Design review of the part built by this model. Coordinates are the model's own, in mm. Face numbers are marked on the shaded views. Give positions to 0.01 mm unless a question says otherwise; leave off trailing zeros. Write each loop counter-clockwise with the first axis right and the second up, starting at its lowest first coordinate (ties: lowest second). Pieces come first, ordered by that corner, then holes. Notation, with made-up numbers: M 45,8 L 73,8 A21 ccw 73,44 Z; hole C 17.5,36 d3. An arc over 180 degrees is marked long. Use a Markdown table: item, result. Add a question column.
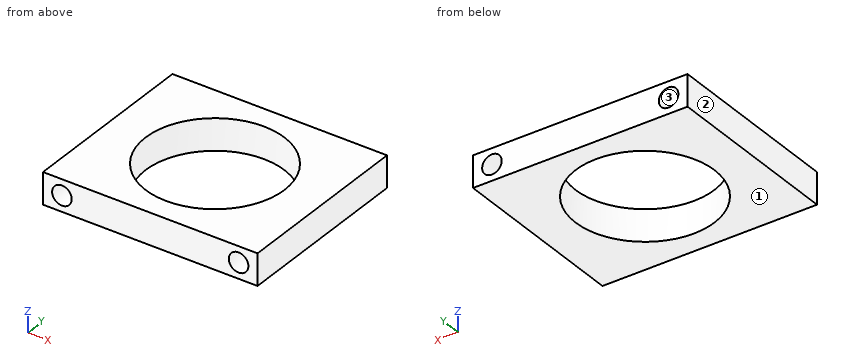
```python
from build123d import *

# Parameters (mm, degrees)
SKETCH_1_W      = 34
SKETCH_1_H      = 29
SKETCH_1_R      = 11
EXTRUDE_1_DEPTH = 5
HOLE_WIZARD_1_D = 3.1


with BuildPart() as part:
    # 草图1 → 凸台-拉伸1 (new body)
    with BuildSketch(Plane.XY):
        Rectangle(SKETCH_1_W, SKETCH_1_H)
        Circle(SKETCH_1_R, mode=Mode.SUBTRACT)
    extrude(amount=EXTRUDE_1_DEPTH)

    # 孔1 (through all)
    with Locations(Plane(origin=(0, 14.5, 0), x_dir=(1, 0, 0), z_dir=(0, 1, 0))):
        with Locations((-14, -2.5), (14, -2.5)):
            Hole(HOLE_WIZARD_1_D / 2)


solid = part.part
```
(1) Wall thickness on L1, parallel to X at y = -1.75, z = 1.3; L2, parallel to X at y = -1.25, z = 1.75; L3, parallel to Z at x = 14, y = 12.5: over which ranges is each line inside the solid? List them lowest first.
(2) The part is to be moulded in two halves that separate along Z. For the marked faces 1, 2 and 3, say which applies: released by +Z, released by -Z, zero draft, split by the parting line, or undercut.
(3) Add section B-B on x = 0. Give the boundary of the cut face in (y, z).
(4) Add section A-A on z = 2.5. Give the boundary of the cut face in (x, y).
(5) Add section D-D on y = 3.5. Give the boundary of the cut face in (x, z), then the cut area to 3 significant figures.
(6) Add section C-C on y = 0. Give the boundary of the cut face in (x, z), then the cut area to 3 significant figures.
(7) For pin 1 (6 mm diameter, centred on x = 3, y = -9.5, fed in from +Z); pin 2 (1.9 mm diameter, centred on x = -14, z = 2.5, fed in from -Y), all flat-tipped, find the tip position at first contact; note any pin that passes through.
From the geometry:
| question | item | result |
|---|---|---|
| 1 | L1 | x = -17 to -14.98, -13.02 to -10.86, 10.86 to 13.02, 14.98 to 17 |
| 1 | L2 | x = -17 to -15.36, -12.64 to -10.93, 10.93 to 12.64, 15.36 to 17 |
| 1 | L3 | z = 0 to 0.95, 4.05 to 5 |
| 2 | face 1 | released by -Z |
| 2 | face 2 | zero draft |
| 2 | face 3 | undercut |
| 3 | outline | M -14.5,0 L -11,0 L -11,5 L -14.5,5 Z; M 11,0 L 14.5,0 L 14.5,5 L 11,5 Z |
| 4 | outline | M -17,-14.5 L -15.55,-14.5 L -15.55,14.5 L -17,14.5 Z; M -12.45,-14.5 L 12.45,-14.5 L 12.45,14.5 L -12.45,14.5 Z; M 15.55,-14.5 L 17,-14.5 L 17,14.5 L 15.55,14.5 Z; hole C 0,0 d22 |
| 5 | outline | M -17,0 L -10.43,0 L -10.43,5 L -17,5 Z; M 10.43,0 L 17,0 L 17,5 L 10.43,5 Z; hole C -14,2.5 d3.1; hole C 14,2.5 d3.1 |
| 5 | area | 50.6 mm^2 |
| 6 | outline | M -17,0 L -11,0 L -11,5 L -17,5 Z; M 11,0 L 17,0 L 17,5 L 11,5 Z; hole C -14,2.5 d3.1; hole C 14,2.5 d3.1 |
| 6 | area | 44.9 mm^2 |
| 7 | pin 1 | stops at z = 5 |
| 7 | pin 2 | passes through |
